```python
from build123d import *

# Parameters (mm, degrees)
ESBO_O1_R                  = 1.6
RESSALTO_EXTRUS_O10_DEPTH  = 3
FILETE2_R                  = 1
CHANFRO1_SIZE              = 1.35
ESBO_O5_W                  = 50
ESBO_O5_H                  = 13
RESSALTO_EXTRUS_O13_DEPTH  = 3
ESBO_O7_R                  = 1.65
CORTE_EXTRUS_O1_DEPTH      = 1
CORTE_EXTRUS_O1_DEPTH_BACK = 4
ESBO_O8_W                  = 10
ESBO_O8_H                  = 15
CORTE_EXTRUS_O2_DEPTH      = 4
FILETE3_R                  = 3
ESBO_O9_R                  = 4
RESSALTO_EXTRUS_O14_DEPTH  = 8
ESBO_O10_R                 = 1.65
CORTE_EXTRUS_O5_DEPTH      = 9


with BuildPart() as part:
    # Esboço1 → Ressalto-extrusão10 (new body)
    with BuildSketch(Plane(origin=(0, 0, 0), x_dir=(1, 0, 0), z_dir=(0, 1, 0))):
        with BuildLine():
            Line((25, 20), (-25, 20))
            Line((-25, 20), (-25, -20))
            Line((-25, -20), (25, -20))
            Line((25, -20), (25, -3.31662479))
            ThreePointArc((25, -3.31662479), (14, 0), (25, 3.31662479))
            Line((25, 3.31662479), (25, 20))
        make_face()
        with Locations((20, -9)):
            Circle(ESBO_O1_R, mode=Mode.SUBTRACT)
        with Locations((20, 9)):
            Circle(ESBO_O1_R, mode=Mode.SUBTRACT)
    extrude(amount=RESSALTO_EXTRUS_O10_DEPTH)

    # Filete2
    filete2_edges = [part.edges().sort_by_distance(p)[0] for p in [
        (25, 1.5, 3.31662479),
        (25, 1.5, -3.31662479),
    ]]
    fillet(filete2_edges, radius=FILETE2_R)

    # Chanfro1
    chanfro1_edges = [part.edges().sort_by_distance(p)[0] for p in [
        (18.4, 0, -9),
        (18.4, 0, 9),
    ]]
    chamfer(chanfro1_edges, length=CHANFRO1_SIZE)

    # Esboço5 → Ressalto-extrusão13 (add)
    with BuildSketch(Plane.XZ):
        with Locations((0, 26.5)):
            Rectangle(ESBO_O5_W, ESBO_O5_H)
    extrude(amount=-RESSALTO_EXTRUS_O13_DEPTH)

    # Esboço7 → Corte-extrusão1 (cut, two sides)
    with BuildSketch(Plane.XZ) as corte_extrus_o1_sk:
        with Locations((-15.5, 28.234562647)):
            Circle(ESBO_O7_R)
        with Locations((4.5, 28.234562647)):
            Circle(ESBO_O7_R)
    extrude(amount=CORTE_EXTRUS_O1_DEPTH, mode=Mode.SUBTRACT)
    extrude(corte_extrus_o1_sk.sketch, amount=-CORTE_EXTRUS_O1_DEPTH_BACK, mode=Mode.SUBTRACT)

    # Esboço8 → Corte-extrusão2 (cut, through all)
    with BuildSketch(Plane.XZ):
        Polygon((-25, -20), (-25, 13), (17, -20), align=None)
        with Locations((20, 25.5)):
            Rectangle(ESBO_O8_W, ESBO_O8_H)
    extrude(amount=-CORTE_EXTRUS_O2_DEPTH, mode=Mode.SUBTRACT)

    # Filete3
    filete3_edges = [part.edges().sort_by_distance(p)[0] for p in [
        (25, 1.5, -20),
        (-25, 1.5, 33),
        (-25, 1.5, 13),
        (17, 1.5, -20),
        (15, 1.5, 18),
        (15, 1.5, 33),
        (25, 1.5, 18),
    ]]
    fillet(filete3_edges, radius=FILETE3_R)

    # Esboço9 → Ressalto-extrusão14 (add)
    with BuildSketch(Plane.XZ):
        with Locations((-15.5, 28.234562647)):
            Circle(ESBO_O9_R)
        with Locations((4.5, 28.234562647)):
            Circle(ESBO_O9_R)
        with Locations((-5.5, 10.234562647)):
            Circle(ESBO_O9_R)
    extrude(amount=RESSALTO_EXTRUS_O14_DEPTH)

    # Esboço10 → Corte-extrusão5 (cut, through all)
    with BuildSketch(Plane.XZ):
        with Locations((-15.5, 28.234562647)):
            Circle(ESBO_O10_R)
        with Locations((4.5, 28.234562647)):
            Circle(ESBO_O10_R)
    extrude(amount=CORTE_EXTRUS_O5_DEPTH, mode=Mode.SUBTRACT)


solid = part.part
```
Check sheet for the modelled part. Datum: model origin and axes. Units: mm. A direction names the side the tool comes from. Round coordinates to 2 decimals unless told otherwise and drop trailing zeros. Order: outer loops, then holes, each group sorted by start corner. A loop starts at its lowest first (then second) coordinate and runs counter-clockwise, first axis right, second up. Notation, with made-up numbers: (-3, 36.25) - (37, 36.25) arc R12 ccw to (37, 40.25) - close; hole circle Ø5 at (-6.75, 75.5). An arc over 180 degrees is marked (long way). Write item = value, one per line.
Q1. Section check C-C (x = -15.5). Record the boundary of the cut face in (y, z).
Computed:
outline = (-8, 24.23) - (0, 24.23) - (0, 5.54) - (3, 5.54) - (3, 26.58) - (-8, 26.58) - close; (-8, 29.88) - (3, 29.88) - (3, 33) - (0, 33) - (0, 32.23) - (-8, 32.23) - close
Q2. Section check B-B (z = -9). Record the boundary of the cut face in (x, y), and give its area (3 significant figures).
Computed:
outline = (3, 0) - (17.05, 0) - (18.4, 1.35) - (18.4, 3) - (3, 3) - close; (21.6, 1.35) - (22.95, 0) - (25, 0) - (25, 3) - (21.6, 3) - close
area = 54.6 mm^2
Q3. Section check A-A (x = 20). Record the boundary of the cut face in (y, z), and give its area (3 significant figures).
Computed:
outline = (0, -20) - (3, -20) - (3, -10.6) - (1.35, -10.6) - (0, -11.95) - close; (0, -6.05) - (1.35, -7.4) - (3, -7.4) - (3, -6) - (0, -6) - close; (0, 6) - (3, 6) - (3, 7.4) - (1.35, 7.4) - (0, 6.05) - close; (0, 11.95) - (1.35, 10.6) - (3, 10.6) - (3, 18) - (0, 18) - close
area = 55.2 mm^2
Q4. Go/stop test with flat-tipped pins: pin 1 (4 mm diameter, centred on x = 3.5, z = -5, fed in from -Y); pin 2 (1.5 mm diameter, centred on x = 20, y = 1.5, fed in from +Z); pin 3 (1.5 mm diameter, centred on y = 1, z = 25, fed in from +X). Record where each tip stops, or that it passes through.
Computed:
pin_1 = 0
pin_2 = 18
pin_3 = 15
Q5. Tool access check on faces 1 (the face through (-24.14, 1.52, 32.1)), 2 (the face through (15, 1, 25)), 3 (the face through (24.476, 1.521, -4.865)), 4 (the face through (-6.02, -3.94, 14.2)). Record the directions out of +Z, -Z, +X, -X, +Y, -Y that give a thin tool (end or side, any length) a straight path to the whole face; none if there is none.
Computed:
face_1 = +Z, -X, +Y, -Y
face_2 = +Z, +X, +Y, -Y
face_3 = +Y, -Y
face_4 = -Y
Q6. Draft check along X on faces 5 (the face through (24.14, 1.52, -19.1)), 6 (the face through (6, -8, 27)), 7 (the face through (-18.674, -3.944, 25.801)), 8 (the face through (17.04, 1.52, -19.83)). Enter one of: pulls with the +X half, pulls with the -X half, needs draft (parallel to the pull), parting line crosses it, or undercut.
Computed:
face_5 = pulls with the +X half
face_6 = needs draft
face_7 = undercut
face_8 = pulls with the -X half
Q7. Thickness scan on line 1 along Z through (x, y) = (20, 2.4); line 2 along Z through (x, y) = (4.5, -2.5); line 3 along Y through (x, z) = (-3, 15). Record the ranges inside material, lowest first.
Computed:
line_1 = -20 to -10.6, -7.4 to -6, 6 to 7.4, 10.6 to 18
line_2 = 24.23 to 26.58, 29.88 to 32.23
line_3 = 0 to 3
Q8. Section check D-D (y = -7). Record the boundary of the cut face in (x, z), and give its area (3 significant figures).
Computed:
outline = circle Ø8 at (-15.5, 28.23); circle Ø8 at (-5.5, 10.23); circle Ø8 at (4.5, 28.23); hole circle Ø3.3 at (-15.5, 28.23); hole circle Ø3.3 at (4.5, 28.23)
area = 134 mm^2
